Geometry: final body of the model. Coordinates: model frame, mm. Give positions to 0.01 mm unless a question says otherwise; leave off trailing zeros. Loops run counter-clockwise (first coordinate to the right, second up) from the corner with the lowest first, then second, coordinate; pieces in that order, holes last. Notation, with made-up numbers: (55.5, 54.5) -> (102.5, 54.5) arc R10 cw to (102.5, 62.5) -> close; hole circle Ø3 at (-17.5, -0.5). An arc over 180 degrees is marked (long way). One line per question, with ' | ' between items. Start each with the question number.
Item 1: Section A-A on z = 2.5. Return loops of the section in (x, y), then the cut area to 3 significant figures.
Item 2: Section C-C on z = 9.5. Return loops of the section in (x, y), then the cut area to 3 significant figures.
Item 3: Material intervals for line 1 along Y through (x, z) = (1.1, 9.5); line 2 along X through (y, z) = (1.5, 10.25); line 3 along X through (y, z) = (2.6, 1.75), sorted ascending. Write a range as [from, to].
Item 4: Section B-B on y = 4.27. Return loops of the section in (x, z).
Item 5: Section D-D on x = 1.27. Return loops of the section in (y, z).
from build123d import *

# Parameters (mm, degrees)
SKETCH_1_W          = 2.54
SKETCH_1_H          = 6
EXTRUDE_1_DEPTH     = 12
SKETCH_2_W          = 2
SKETCH_2_H          = 2
CUT_EXTRUDE_1_DEPTH = 4
SKETCH_3_R          = 0.65
EXTRUDE_2_DEPTH     = 4
SKETCH_4_W          = 0.8
SKETCH_4_H          = 0.8
CUT_EXTRUDE_2_DEPTH = 5


with BuildPart() as part:
    # Эскиз1 → Бобышка-Вытянуть1 (new body)
    with BuildSketch(Plane.XY):
        with Locations((1.27, 3)):
            Rectangle(SKETCH_1_W, SKETCH_1_H)
    extrude(amount=EXTRUDE_1_DEPTH)

    # Эскиз2 → Вырез-Вытянуть1 (cut)
    with BuildSketch(Plane(origin=(0, 0, 0), x_dir=(-1, 0, 0), z_dir=(0, 0, -1))):
        with Locations((-1.27, 4.27)):
            Rectangle(SKETCH_2_W, SKETCH_2_H)
        with Locations((-1.27, 1.73)):
            Rectangle(SKETCH_2_W, SKETCH_2_H)
    extrude(amount=-CUT_EXTRUDE_1_DEPTH, mode=Mode.SUBTRACT)

    # Эскиз3 → Бобышка-Вытянуть2 (add)
    with BuildSketch(Plane(origin=(0, 0, 4), x_dir=(-1, 0, 0), z_dir=(0, 0, -1))):
        with Locations((-1.27, 4.27)):
            Circle(SKETCH_3_R)
        with Locations((-1.27, 1.73)):
            Circle(SKETCH_3_R)
    extrude(amount=EXTRUDE_2_DEPTH)

    # Эскиз4 → Вырез-Вытянуть2 (cut)
    with BuildSketch(Plane.XY.offset(12)):
        with Locations((1.27, 4.27)):
            Rectangle(SKETCH_4_W, SKETCH_4_H)
        with Locations((1.27, 1.73)):
            Rectangle(SKETCH_4_W, SKETCH_4_H)
    extrude(amount=-CUT_EXTRUDE_2_DEPTH, mode=Mode.SUBTRACT)


solid = part.part
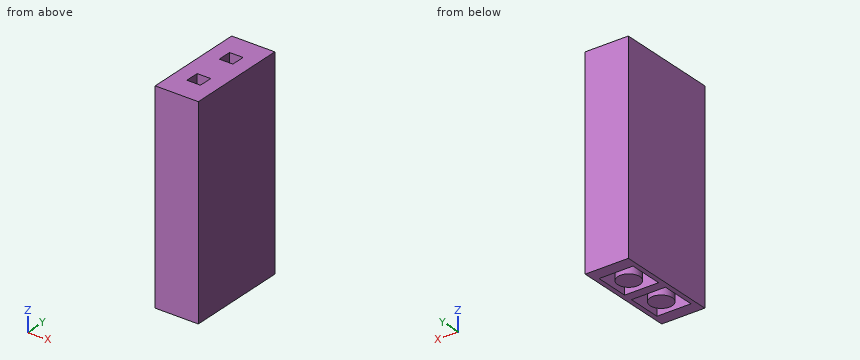
Result sheet:
1) outline: (0, 0) -> (2.54, 0) -> (2.54, 6) -> (0, 6) -> close; circle Ø1.3 at (1.27, 1.73); circle Ø1.3 at (1.27, 4.27); hole (0.27, 0.73) -> (2.27, 0.73) -> (2.27, 2.73) -> (0.27, 2.73) -> close; hole (0.27, 3.27) -> (2.27, 3.27) -> (2.27, 5.27) -> (0.27, 5.27) -> close | area: 9.89 mm²
2) outline: (0, 0) -> (2.54, 0) -> (2.54, 6) -> (0, 6) -> close; hole (0.87, 1.33) -> (1.67, 1.33) -> (1.67, 2.13) -> (0.87, 2.13) -> close; hole (0.87, 3.87) -> (1.67, 3.87) -> (1.67, 4.67) -> (0.87, 4.67) -> close | area: 14.0 mm²
3) line 1: y = [0, 1.33], [2.13, 3.87], [4.67, 6] | line 2: x = [0, 0.87], [1.67, 2.54] | line 3: x = [0, 0.27], [2.27, 2.54]
4) outline: (0, 0) -> (0.27, 0) -> (0.27, 4) -> (0.62, 4) -> (0.62, 0) -> (1.92, 0) -> (1.92, 4) -> (2.27, 4) -> (2.27, 0) -> (2.54, 0) -> (2.54, 12) -> (1.67, 12) -> (1.67, 7) -> (0.87, 7) -> (0.87, 12) -> (0, 12) -> close
5) outline: (0, 0) -> (0.73, 0) -> (0.73, 4) -> (1.08, 4) -> (1.08, 0) -> (2.38, 0) -> (2.38, 4) -> (2.73, 4) -> (2.73, 0) -> (3.27, 0) -> (3.27, 4) -> (3.62, 4) -> (3.62, 0) -> (4.92, 0) -> (4.92, 4) -> (5.27, 4) -> (5.27, 0) -> (6, 0) -> (6, 12) -> (4.67, 12) -> (4.67, 7) -> (3.87, 7) -> (3.87, 12) -> (2.13, 12) -> (2.13, 7) -> (1.33, 7) -> (1.33, 12) -> (0, 12) -> close
